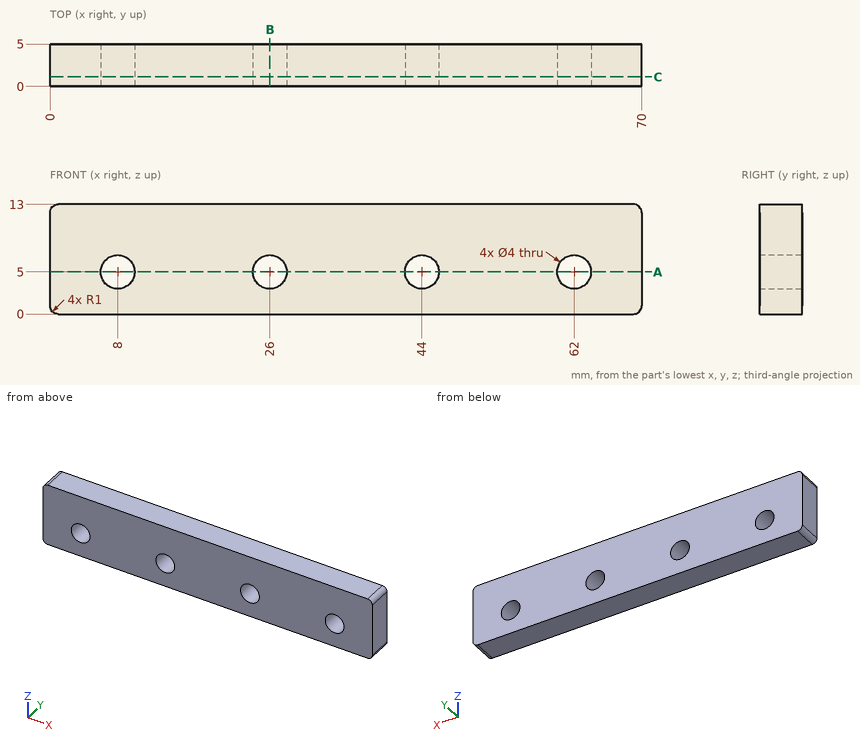
Geometry check sheet. Reference: drawing and pictorial views, mm from the part's lowest x, y, z. Give positions to 0.01 mm unless a question says otherwise; leave off trailing zeros. Order: outer loops, then holes, each group sorted by start corner. A loop starts at its lowest first (then second) coordinate and runs counter-clockwise, first axis right, second up. Notation, with made-up numbers: M 49.5,61 L 69.5,61 A23 ccw 69.5,81 Z; hole C 23,38 d2. An arc over 180 degrees is marked long. Answer in a Markdown table with one row per item. Add a question column.
Item 1: Section check A-A, the plane z = 5. Enter the section's corners in (x, y).
Item 2: Section check B-B, the plane x = 26. Enter the section's corners in (y, z), and give its area (3 significant figures).
Item 3: Section check C-C, the plane y = 1.1. Enter the section's corners in (x, z).
Item 4: Gauge pin test, flat end, axial feed: pin 1 (1 mm diameter, centred on x = 63, z = 4.5, fed in from -Y). Record the tip position at first contact, or that the pin passes through.
Item 5: Scan lines: probe 1 along X at (y, z) = (1.65, 5); probe 2 along X at (y, z) = (1.65, 4.5); probe 3 along Z at (x, y) = (62, 1.2). Record each from-to range of solid material in increasing order. Write a range as from..to.
Filled sheet:
| question | item | result |
|---|---|---|
| 1 | outline | M 0,0 L 6,0 L 6,5 L 0,5 Z; M 10,0 L 24,0 L 24,5 L 10,5 Z; M 28,0 L 42,0 L 42,5 L 28,5 Z; M 46,0 L 60,0 L 60,5 L 46,5 Z; M 64,0 L 70,0 L 70,5 L 64,5 Z |
| 2 | outline | M 0,0 L 5,0 L 5,3 L 0,3 Z; M 0,7 L 5,7 L 5,13 L 0,13 Z |
| 2 | area | 45.0 mm^2 |
| 3 | outline | M 0,1 A1 ccw 1,0 L 69,0 A1 ccw 70,1 L 70,12 A1 ccw 69,13 L 1,13 A1 ccw 0,12 Z; hole C 8,5 d4; hole C 26,5 d4; hole C 44,5 d4; hole C 62,5 d4 |
| 4 | pin 1 | passes through |
| 5 | probe 1 | x = 0..6, 10..24, 28..42, 46..60, 64..70 |
| 5 | probe 2 | x = 0..6.06, 9.94..24.06, 27.94..42.06, 45.94..60.06, 63.94..70 |
| 5 | probe 3 | z = 0..3, 7..13 |
